```python
from build123d import *

# Parameters (mm, degrees)
EXTRUDE_1_DEPTH      = 5
SKETCH_9_R           = 1.5
CUT_EXTRUDE_7_DEPTH  = 5
SKETCH_7_R           = 2.1
CUT_EXTRUDE_8_DEPTH  = 5
CUT_EXTRUDE_9_REACH  = 335.054
SKETCH_10_W          = 60
SKETCH_10_H          = 90
CUT_EXTRUDE_11_REACH = 335.054


with BuildPart() as part:
    # 草图1 → 凸台-拉伸1 (new body)
    with BuildSketch(Plane.XY):
        with BuildLine():
            Line((10, 0), (240, 0))
            ThreePointArc((240, 0), (247.071067812, -2.928932188), (250, -10))
            Line((250, -10), (250, -210))
            ThreePointArc((250, -210), (247.071067812, -217.071067812), (240, -220))
            Line((240, -220), (10, -220))
            ThreePointArc((10, -220), (2.928932188, -217.071067812), (0, -210))
            Line((0, -210), (0, -10))
            ThreePointArc((0, -10), (2.928932188, -2.928932188), (10, 0))
        make_face()
    extrude(amount=EXTRUDE_1_DEPTH)

    # 草图9 → 切除-拉伸7 (cut)
    with BuildSketch(Plane.XY.offset(5)):
        with Locations((40, -10)):
            Circle(SKETCH_9_R)
        with Locations((125, -10)):
            Circle(SKETCH_9_R)
        with Locations((210, -10)):
            Circle(SKETCH_9_R)
    extrude(amount=-CUT_EXTRUDE_7_DEPTH, mode=Mode.SUBTRACT)

    # 草图7 → 切除-拉伸8 (cut)
    with BuildSketch(Plane(origin=(0, 0, 0), x_dir=(-1, 0, 0), z_dir=(0, 0, -1))):
        with Locations((-74.4, -40)):
            Circle(SKETCH_7_R)
        with Locations((-35.6, -40)):
            Circle(SKETCH_7_R)
        with Locations(Location((-214.4, -40, 0), (0, 0, 180))):
            Circle(SKETCH_7_R)
        with Locations(Location((-175.6, -40, 0), (0, 0, 180))):
            Circle(SKETCH_7_R)
    extrude(amount=-CUT_EXTRUDE_8_DEPTH, mode=Mode.SUBTRACT)

    # 草图10 → 切除-拉伸9 (cut, up to next)
    with BuildSketch(Plane.XY.offset(5), mode=Mode.PRIVATE) as cut_extrude_9_sk1:
        with Locations((220, -175)):
            Rectangle(SKETCH_10_W, SKETCH_10_H)
    cut_extrude_9_tool1 = extrude(cut_extrude_9_sk1.sketch, amount=-CUT_EXTRUDE_9_REACH, mode=Mode.PRIVATE) & part.part
    # 草图10 → 切除-拉伸9 (cut, up to next)
    with BuildSketch(Plane.XY.offset(5), mode=Mode.PRIVATE) as cut_extrude_9_sk2:
        with Locations((30, -175)):
            Rectangle(SKETCH_10_W, SKETCH_10_H)
    cut_extrude_9_tool2 = extrude(cut_extrude_9_sk2.sketch, amount=-CUT_EXTRUDE_9_REACH, mode=Mode.PRIVATE) & part.part
    add(cut_extrude_9_tool1.solids().sort_by_distance((220, -175, 5))[0], mode=Mode.SUBTRACT)
    add(cut_extrude_9_tool2.solids().sort_by_distance((30, -175, 5))[0], mode=Mode.SUBTRACT)

    # 草图11 → 切除-拉伸11 (cut, up to next)
    with BuildSketch(Plane.XY.offset(5), mode=Mode.PRIVATE) as cut_extrude_11_sk1:
        with BuildLine():
            Line((0, -130), (10, -130))
            ThreePointArc((10, -130), (2.928932188, -127.071067812), (0, -120))
            Line((0, -120), (0, -130))
        make_face()
    cut_extrude_11_tool1 = extrude(cut_extrude_11_sk1.sketch, amount=-CUT_EXTRUDE_11_REACH, mode=Mode.PRIVATE) & part.part
    # 草图11 → 切除-拉伸11 (cut, up to next)
    with BuildSketch(Plane.XY.offset(5), mode=Mode.PRIVATE) as cut_extrude_11_sk2:
        with BuildLine():
            ThreePointArc((70, -220), (62.928932188, -217.071067812), (60, -210))
            Line((60, -210), (60, -220))
            Line((60, -220), (70, -220))
        make_face()
    cut_extrude_11_tool2 = extrude(cut_extrude_11_sk2.sketch, amount=-CUT_EXTRUDE_11_REACH, mode=Mode.PRIVATE) & part.part
    # 草图11 → 切除-拉伸11 (cut, up to next)
    with BuildSketch(Plane.XY.offset(5), mode=Mode.PRIVATE) as cut_extrude_11_sk3:
        with BuildLine():
            ThreePointArc((190, -210), (187.071067812, -217.071067812), (180, -220))
            Line((180, -220), (190, -220))
            Line((190, -220), (190, -210))
        make_face()
    cut_extrude_11_tool3 = extrude(cut_extrude_11_sk3.sketch, amount=-CUT_EXTRUDE_11_REACH, mode=Mode.PRIVATE) & part.part
    # 草图11 → 切除-拉伸11 (cut, up to next)
    with BuildSketch(Plane.XY.offset(5), mode=Mode.PRIVATE) as cut_extrude_11_sk4:
        with BuildLine():
            ThreePointArc((250, -120), (247.071067812, -127.071067812), (240, -130))
            Line((240, -130), (250, -130))
            Line((250, -130), (250, -120))
        make_face()
    cut_extrude_11_tool4 = extrude(cut_extrude_11_sk4.sketch, amount=-CUT_EXTRUDE_11_REACH, mode=Mode.PRIVATE) & part.part
    add(cut_extrude_11_tool1.solids().sort_by_distance((2.233679, -127.766321, 5))[0], mode=Mode.SUBTRACT)
    add(cut_extrude_11_tool2.solids().sort_by_distance((62.233679, -217.766321, 5))[0], mode=Mode.SUBTRACT)
    add(cut_extrude_11_tool3.solids().sort_by_distance((187.766321, -217.766321, 5))[0], mode=Mode.SUBTRACT)
    add(cut_extrude_11_tool4.solids().sort_by_distance((247.766321, -127.766321, 5))[0], mode=Mode.SUBTRACT)


solid = part.part
```
Geometry check sheet. Reference: the model listing, model coordinates, mm. A direction names the side the tool comes from. Coordinates: 2 decimals unless noted, no trailing zeros. Loops run counter-clockwise (first coordinate to the right, second up) from the corner with the lowest first, then second, coordinate; pieces in that order, holes last. Notation, with made-up numbers: (19.25, 55) - (78.25, 55) arc R15 ccw to (78.25, 73) - close; hole circle Ø3 at (64.25, -18). An arc over 180 degrees is marked (long way). One line per item, written item: value. Start each with the question number.
(1) Cross-section at B-B on x = 204. Enter the section's corners in (y, z), plus the area to 3 significant figures.
(2) Tool access check on faces 1 (the flat face through (190, -171, 3)), 2 (the flat face through (123, 0, 2)), 3 (the flat face through (60, -171, 3)). Record the directions out of +Z, -Z, +X, -X, +Y, -Y that give a thin tool (end or side, any length) a straight path to the whole face; none if there is none.
(3) Depth check by flat-ended pin: P1, Ø3, axis at y = -127, z = 4.5, coming from the +X side; P2, Ø2.5, axis at x = 45.5, z = 3.5, coming from the -Y side. Enter the tip coordinate at first touch or a pass-through.
(4) Material ranges on line 1 (Y direction, x = 40, z = 2.8); line 2 (Y direction, x = 74.4, z = 3.4); line 3 (X direction, y = -174.5, z = 1.25), recorded low to high. Write a range as [from, to].
(5) Cross-section at A-A on z = 2.95. Enter the section's corners in (x, y), plus the area to 3 significant figures.
(6) Cross-section at C-C on y = -154. Enter the section's corners in (x, z), plus the area to 3 significant figures.
Results below:
1. outline: (-130, 0) - (0, 0) - (0, 5) - (-130, 5) - close
1. area: 650 mm2
2. face 1: +Z, -Z, +X, -Y
2. face 2: +Z, -Z, +X, -X, +Y
2. face 3: +Z, -Z, -X, -Y
3. P1: stops at x = 248.35
3. P2: stops at y = -130
4. line 1: y = [-130, -11.5], [-8.5, 0]
4. line 2: y = [-220, -42.1], [-37.9, 0]
4. line 3: x = [60, 190]
5. outline: (0, -120) arc R10 ccw to (10, -130) - (60, -130) - (60, -210) arc R10 ccw to (70, -220) - (180, -220) arc R10 ccw to (190, -210) - (190, -130) - (240, -130) arc R10 ccw to (250, -120) - (250, -10) arc R10 ccw to (240, 0) - (10, 0) arc R10 ccw to (0, -10) - close; hole circle Ø4.2 at (35.6, -40); hole circle Ø3 at (40, -10); hole circle Ø4.2 at (74.4, -40); hole circle Ø3 at (125, -10); hole circle Ø4.2 at (175.6, -40); hole circle Ø3 at (210, -10); hole circle Ø4.2 at (214.4, -40)
5. area: 44,000 mm2
6. outline: (60, 0) - (190, 0) - (190, 5) - (60, 5) - close
6. area: 650 mm2
